Autodesk Inventor part; units mm, degrees
ref_plane "YZ Plane" through (0, 0, 0) normal (1, 0, 0) x (0, 1, 0)
ref_plane "XZ Plane" through (0, 0, 0) normal (0, 1, 0) x (-1, 0, 0)
ref_plane "XY Plane" through (0, 0, 0) normal (0, 0, 1) x (1, 0, 0)
sketch "Sketch1" plane through (0, 0, 0) normal (0, 1, 0) x (-1, 0, 0)
  line L0 (0, 0) -> (-17.78, 0)
  line L1 (-17.78, 0) -> (-17.78, -44.45)
  line L2 (-17.78, -44.45) -> (0, -44.45)
  line L3 (0, -44.45) -> (0, 0)
  line L4 (-17.78, -44.45) -> (-35.56, -44.45)
  line L5 (-35.56, -44.45) -> (-35.56, -31.75)
  line L6 (-35.56, -31.75) -> (-17.78, -31.75)
  line L7 (-17.78, -31.75) -> (-17.78, -44.45)
  dimension "d0" = 17.78
  dimension "d1" = 44.45
  dimension "d2" = 17.78
  dimension "d3" = 12.7
extrude "Extrusion1" add sketch "Sketch1" along normal blind 18.288
sketch "Sketch2" plane through (17.78, 0, -31.75) normal (0, 0, 1) x (1, 0, 0)
  circle A0 centre (9.4883, 9.144) radius 6.35
  point P0 (-17.78, 0)
  dimension "d6" = 12.7
extrude "Extrusion2" cut sketch "Sketch2" against normal blind 12.7
sketch "Sketch3" plane through (0, 18.288, 0) normal (0, 1, 0) x (1, 0, 0)
  circle A0 centre (8.89, 8.89) radius 6.35
  line L0 (0, 0) -> (17.78, 0)
  dimension "d9" = 12.7
  dimension "d10" = 8.89
extrude "Extrusion3" cut sketch "Sketch3" against normal blind 18.288
properties part number "Pivot Point 2"
Input: part model. Units: mm. Frame: model coordinates. A direction names the side the tool comes from. Round coordinates to 2 decimals unless told otherwise and drop trailing zeros. Loops run counter-clockwise (first coordinate to the right, second up) from the corner with the lowest first, then second, coordinate; pieces in that order, holes last. Notation, with made-up numbers: (-25, 18.25) -> (19, 18.25) arc R24 cw to (19, 49.25) -> close; hole circle Ø11 at (-16, 51.5). An arc over 180 degrees is marked (long way). Use one line per item in the form item = value. Start each with the question number.
Item 1: Section query C-C on z = -8.89. Return the cut outline in (x, y).
Item 2: Contact query for flat-ended pins moving along their axis: pin 1 Ø2 at (y, z) = (3, -32.5) entering from -X; pin 2 Ø4 at (y, z) = (3.5, -4.5) entering from +X; pin 3 Ø5 at (x, z) = (20.5, -6) entering from +Y; pin 4 Ø6 at (x, y) = (22, 9.5) entering from +Z. Output: stop coordinate, or through.
Item 3: Section query B-B on x = 8.89. Return the cut outline in (y, z).
Item 4: Mould query, pull axis Z, two halves, no side actions, for faces 1 (the face through (35.56, 9, -38)), 2 (the face through (18, 9, -44.45)), 3 (the face through (21, 7, -31.75)), 4 (the face through (7.51, 9.27, -2.69)). Classes: pulls with the +Z half, pulls with the -Z half, needs draft (parallel to the pull), parting line crosses it, or undercut.
Item 5: Material intervals for L1, parallel to Z at x = 8.89, y = 13.75; L2, parallel to X at y = 4.5, z = -8.89; L3, parallel to X at y = 3, z = -8.5, sorted ascending. Write a range as from..to.
Item 6: Set-up query: faces 5 (the face through (14, 0, -27)), 6 (the face through (17.78, 9, -16)). Return all of +Z, -Z, +X, -X, +Y, -Y with unobstructed straight access to the full face (end or side cutting, diameter ignored); none if empty.
Item 7: Section query A-A on y = 8.5. Return the cut outline in (x, z).
Ans:
q1.outline = (0, 0) -> (2.54, 0) -> (2.54, 18.29) -> (0, 18.29) -> close; (15.24, 0) -> (17.78, 0) -> (17.78, 18.29) -> (15.24, 18.29) -> close
q2.pin_1 = 0
q2.pin_2 = 17.78
q2.pin_3 = through
q2.pin_4 = -31.75
q3.outline = (0, -44.45) -> (18.29, -44.45) -> (18.29, -15.24) -> (0, -15.24) -> close; (0, -2.54) -> (18.29, -2.54) -> (18.29, 0) -> (0, 0) -> close
q4.face_1 = needs draft
q4.face_2 = pulls with the -Z half
q4.face_3 = pulls with the +Z half
q4.face_4 = undercut
q5.L1 = -44.45..-15.24, -2.54..0
q5.L2 = 0..2.54, 15.24..17.78
q5.L3 = 0..2.55, 15.23..17.78
q6.face_5 = +Z, -Z, +X, -X, -Y
q6.face_6 = +Z, +X, +Y, -Y
q7.outline = (0, -44.45) -> (20.95, -44.45) -> (20.95, -31.75) -> (17.78, -31.75) -> (17.78, 0) -> (0, 0) -> close; (33.59, -44.45) -> (35.56, -44.45) -> (35.56, -31.75) -> (33.59, -31.75) -> close; hole circle Ø12.7 at (8.89, -8.89)
